Geometry: final body of the model. Coordinates: model frame, mm. Face numbers are marked on the shaded views. A direction names the side the tool comes from. Give positions to 0.01 mm unless a question says otherwise; leave off trailing zeros. Order: outer loops, then holes, each group sorted by start corner. A loop starts at its lowest first (then second) coordinate and runs counter-clockwise, first axis right, second up. Notation, with made-up numbers: (45.25, -25) -> (56.25, -25) arc R16 ccw to (56.25, -1) -> close; hole circle Ø10 at (37, 1). An arc over 180 degrees is marked (long way). Answer in a Markdown table with one row per item. Add a question column.
Q1. Contact query for flat-ended pins moving along their axis: P1, Ø23.5, axis at x = 40, y = 515, coming from the -Z side; P2, Ø5, axis at y = 100.5, z = 34, coming from the +X side; P3, Ø6, axis at y = 375.5, z = 5, coming from the -X side; P4, Ø3, axis at x = 759.5, y = 474.5, coming from the +Z side. Output: stop coordinate, or through.
Q2. Cut plane B-B on y = 75. Return the cut outline in (x, z).
Q3. Cut plane A-A on x = 40. Count the separate pieces of the cut face and the enclosed holes in it, and give its area (3 significant figures).
Q4. Cut plane D-D on y = 261. Return the cut outline in (x, z), and give its area (3 significant figures).
Q5. Pull-direction query (Y, two-part tool) for the marked faces 1, 2 and 3; classes: +Y half, -Y half, draft (parallel to the pull), parting line (faces both ways), or undercut.
Q6. Line query: line 1 along X through (y, z) = (515, 3); line 2 along X through (y, z) = (436, 25.5); line 3 along Y through (x, z) = (235, 74). Output: solid intervals per line, ascending. Write a range as from..to.
Q7. Cut plane C-C on z = -21.5. Return the cut outline in (x, y).
Q8. Set-up query: the marked faces 4, 5, 6, 7 and 8. Return all of +Z, -Z, +X, -X, +Y, -Y with unobstructed straight access to the full face (end or side cutting, diameter ignored); none if empty.
from build123d import *

# Parameters (mm, degrees)
SKETCH_1_W          = 960
SKETCH_1_H          = 550
EXTRUDE_1_DEPTH     = 12
SKETCH_2_W          = 640
SKETCH_2_H          = 162.5
EXTRUDE_2_DEPTH     = 12
SKETCH_3_W          = 640
SKETCH_3_H          = 162.5
EXTRUDE_3_DEPTH     = 12
SKETCH_4_W          = 12.5
SKETCH_4_H          = 526
EXTRUDE_4_DEPTH     = 162.5
SKETCH_5_R          = 13
CUT_EXTRUDE_1_DEPTH = 1110.825464882
SKETCH_6_W          = 50
SKETCH_6_H          = 50
CUT_EXTRUDE_2_DEPTH = 1110.825464882


with BuildPart() as part:
    # 草图1 → 凸台-拉伸1 (new body)
    with BuildSketch(Plane.XY):
        with Locations((480, 275)):
            Rectangle(SKETCH_1_W, SKETCH_1_H)
    extrude(amount=EXTRUDE_1_DEPTH)

    # 草图2 → 凸台-拉伸2 (add)
    with BuildSketch(Plane(origin=(0, 550, 0), x_dir=(1, 0, 0), z_dir=(0, 1, 0))):
        with Locations((480, -6)):
            Rectangle(SKETCH_2_W, SKETCH_2_H)
    extrude(amount=-EXTRUDE_2_DEPTH)

    # 草图3 → 凸台-拉伸3 (add)
    with BuildSketch(Plane.XZ):
        with Locations((480, 6)):
            Rectangle(SKETCH_3_W, SKETCH_3_H)
    extrude(amount=-EXTRUDE_3_DEPTH)

    # 草图4 → 凸台-拉伸4 (add)
    with BuildSketch(Plane(origin=(0, 0, -75.25), x_dir=(-1, 0, 0), z_dir=(0, 0, -1))):
        with Locations((-600, 275)):
            Rectangle(SKETCH_4_W, SKETCH_4_H)
        with Locations((-360, 275)):
            Rectangle(SKETCH_4_W, SKETCH_4_H)
    extrude(amount=-EXTRUDE_4_DEPTH)

    # 草图5 → 切除-拉伸1 (cut, through all)
    with BuildSketch(Plane.XY.offset(12)):
        with Locations((40, 515)):
            Circle(SKETCH_5_R)
        with Locations((40, 435)):
            Circle(SKETCH_5_R)
        with Locations((40, 295)):
            Circle(SKETCH_5_R)
        with Locations((40, 35)):
            Circle(SKETCH_5_R)
        with Locations((112, 235)):
            Circle(SKETCH_5_R)
        with Locations((112, 155)):
            Circle(SKETCH_5_R)
        with Locations((112, 475)):
            Circle(SKETCH_5_R)
        with Locations((112, 395)):
            Circle(SKETCH_5_R)
        with Locations((112, 315)):
            Circle(SKETCH_5_R)
        with Locations((112, 75)):
            Circle(SKETCH_5_R)
        with Locations((40, 195)):
            Circle(SKETCH_5_R)
        with Locations((40, 115)):
            Circle(SKETCH_5_R)
        with Locations((160, 295)):
            Circle(SKETCH_5_R)
    cut_extrude_1 = extrude(amount=-CUT_EXTRUDE_1_DEPTH, mode=Mode.SUBTRACT)

    # 镜向1: 切除-拉伸1 across plane
    add(cut_extrude_1.mirror(Plane.ZY.offset(-480)), mode=Mode.SUBTRACT)

    # 草图6 → 切除-拉伸2 (cut, through all)
    with BuildSketch(Plane(origin=(0, 0, 0), x_dir=(-1, 0, 0), z_dir=(0, 0, -1))):
        with Locations((-25, 370)):
            Rectangle(SKETCH_6_W, SKETCH_6_H)
        with Locations((-935, 370)):
            Rectangle(SKETCH_6_W, SKETCH_6_H)
    extrude(amount=-CUT_EXTRUDE_2_DEPTH, mode=Mode.SUBTRACT)


solid = part.part
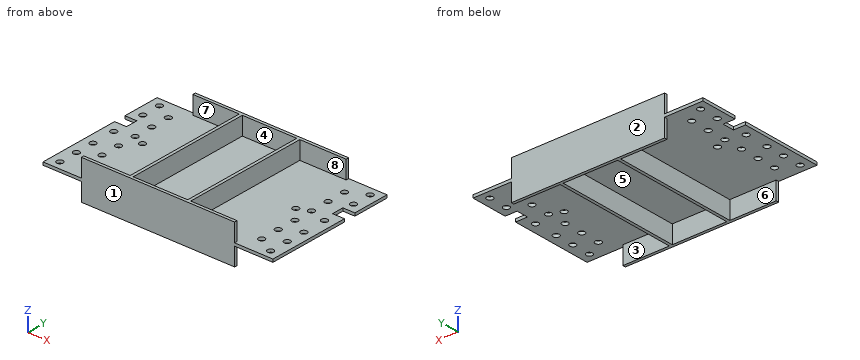
Completed:
| question | item | result |
|---|---|---|
| 1 | P1 | passes through |
| 1 | P2 | stops at x = 606.25 |
| 1 | P3 | stops at x = 50 |
| 1 | P4 | stops at z = 12 |
| 2 | outline | (0, 0) -> (99, 0) -> (99, 12) -> (0, 12) -> close; (125, 0) -> (353.75, 0) -> (353.75, -75.25) -> (366.25, -75.25) -> (366.25, 0) -> (593.75, 0) -> (593.75, -75.25) -> (606.25, -75.25) -> (606.25, 0) -> (835, 0) -> (835, 12) -> (606.25, 12) -> (606.25, 87.25) -> (593.75, 87.25) -> (593.75, 12) -> (366.25, 12) -> (366.25, 87.25) -> (353.75, 87.25) -> (353.75, 12) -> (125, 12) -> close; (861, 0) -> (960, 0) -> (960, 12) -> (861, 12) -> close |
| 3 | separate pieces | 8 |
| 3 | enclosed holes | 0 |
| 3 | area | 4,130 mm² |
| 4 | outline | (0, 0) -> (353.75, 0) -> (353.75, -75.25) -> (366.25, -75.25) -> (366.25, 0) -> (593.75, 0) -> (593.75, -75.25) -> (606.25, -75.25) -> (606.25, 0) -> (960, 0) -> (960, 12) -> (606.25, 12) -> (606.25, 87.25) -> (593.75, 87.25) -> (593.75, 12) -> (366.25, 12) -> (366.25, 87.25) -> (353.75, 87.25) -> (353.75, 12) -> (0, 12) -> close |
| 4 | area | 15,300 mm² |
| 5 | face 1 | -Y half |
| 5 | face 2 | +Y half |
| 5 | face 3 | undercut |
| 6 | line 1 | x = 0..27, 53..907, 933..960 |
| 6 | line 2 | x = 353.75..366.25, 593.75..606.25 |
| 6 | line 3 | y = 0..12, 538..550 |
| 7 | outline | (160, 0) -> (800, 0) -> (800, 12) -> (606.25, 12) -> (606.25, 538) -> (800, 538) -> (800, 550) -> (160, 550) -> (160, 538) -> (353.75, 538) -> (353.75, 12) -> (160, 12) -> close; hole (366.25, 12) -> (593.75, 12) -> (593.75, 538) -> (366.25, 538) -> close |
| 8 | face 4 | +Z |
| 8 | face 5 | -Z |
| 8 | face 6 | -Z, -X |
| 8 | face 7 | +Z, -X |
| 8 | face 8 | +Z, +X |
